For this review, take the finished solid that the model builds, in its own axes (mm). Face numbers are marked on the shaded views. A direction names the side the tool comes from. Round coordinates to 2 decimals unless told otherwise and drop trailing zeros. Write each loop counter-clockwise with the first axis right and the second up, starting at its lowest first coordinate (ties: lowest second). Pieces come first, ordered by that corner, then holes. Notation, with made-up numbers: M -18.5,42.25 L 2.5,42.25 A26 cw 2.5,59.25 Z; hole C -35,-6.5 d7. An arc over 180 degrees is marked long. Answer in a Markdown table with one row per item.
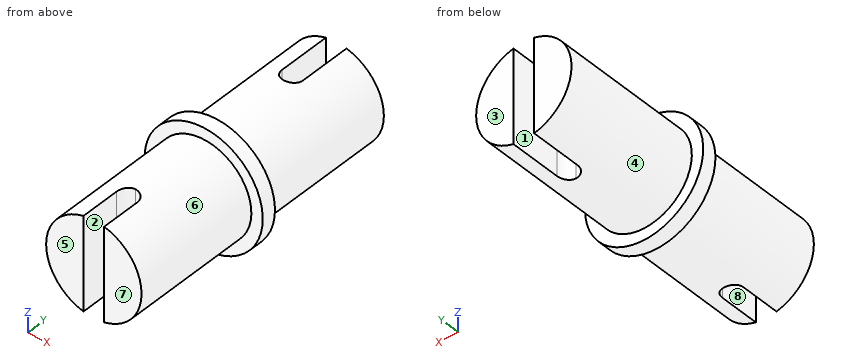
```python
from build123d import *

# Parameters (mm, degrees)
SKETCH2_R            = 2.85
BOSS_EXTRUDE1_DEPTH  = 0.35
SKETCH4_R            = 2.3
BOSS_EXTRUDE2_DEPTH  = 6.9
CUT_EXTRUDE1_START   = -3
CUT_EXTRUDE1_DEPTH   = 3
FILLET1_R            = 0.5
FILLET1_OF_MIRROR1_R = 0.5
CUT_EXTRUDE2_DEPTH   = 0.6


with BuildPart() as part:
    # Sketch2 → Boss-Extrude1 (new body)
    with BuildSketch(Plane(origin=(0, 0, 0), x_dir=(1, 0, 0), z_dir=(0, 1, 0))):
        with Locations(Location((0, 0, 0), (0, 0, 270))):
            Circle(SKETCH2_R)
    boss_extrude1 = extrude(amount=BOSS_EXTRUDE1_DEPTH)

    # Sketch4 → Boss-Extrude2 (add)
    with BuildSketch(Plane(origin=(0, 0.35, 0), x_dir=(1, 0, 0), z_dir=(0, 1, 0))):
        with Locations(Location((0, 0, 0), (0, 0, 90))):
            Circle(SKETCH4_R)
    boss_extrude2 = extrude(amount=BOSS_EXTRUDE2_DEPTH)

    # Sketch5 → Cut-Extrude1 (cut)
    with BuildSketch(Plane(origin=(0, 7.25, 0), x_dir=(1, 0, 0), z_dir=(0, 1, 0)).offset(CUT_EXTRUDE1_START)):
        with BuildLine():
            Line((-0.5, 2.244994432), (-0.5, -2.244994432))
            ThreePointArc((-0.5, -2.244994432), (0, -2.3), (0.5, -2.244994432))
            Line((0.5, -2.244994432), (0.5, 2.244994432))
            ThreePointArc((0.5, 2.244994432), (0, 2.3), (-0.5, 2.244994432))
        make_face()
    cut_extrude1 = extrude(amount=CUT_EXTRUDE1_DEPTH, mode=Mode.SUBTRACT)

    # Fillet1
    fillet1_edges = [part.edges().sort_by_distance(p)[0] for p in [
        (0.5, 4.25, 0),
        (-0.5, 4.25, 0),
    ]]
    fillet(fillet1_edges, radius=FILLET1_R - 0.0001)  # a hair under: the kernel refuses the full size

    # Mirror1: Boss-Extrude1, Boss-Extrude2, Cut-Extrude1 across plane
    add(boss_extrude1.mirror(Plane.ZX))
    add(boss_extrude2.mirror(Plane.ZX))
    add(cut_extrude1.mirror(Plane.ZX), mode=Mode.SUBTRACT)

    # Fillet1 of Mirror1
    fillet1_of_mirror1_edges = [part.edges().sort_by_distance(p)[0] for p in [
        (0.5, -4.25, 0),
        (-0.5, -4.25, 0),
    ]]
    fillet(fillet1_of_mirror1_edges, radius=FILLET1_OF_MIRROR1_R - 0.0001)  # a hair under: the kernel refuses the full size

    # Sketch6 → Cut-Extrude2 (cut)
    with BuildSketch(Plane(origin=(0, -7.25, 0), x_dir=(-1, 0, 0), z_dir=(0, -1, 0))):
        with BuildLine():
            ThreePointArc((0.5, -2.244994432), (2.244994432, 0.5), (-0.5, 2.244994432))
            ThreePointArc((-0.5, 2.244994432), (-2.244994432, -0.5), (0.5, -2.244994432))
        make_face()
    extrude(amount=-CUT_EXTRUDE2_DEPTH, mode=Mode.SUBTRACT)


solid = part.part
```
Q1. For probe 1 along Y at (x, z) = (-1.25, -2.2); probe 2 along X at (y, z) = (-6, -0.45); probe 3 along Z at (x, y) = (-0.1, -2.5), list the stretches that pass through material, from the lowest coordinate up.
Found:
| item | result |
|---|---|
| probe 1 | -0.35 to 0.35 |
| probe 2 | -2.26 to -0.5, 0.5 to 2.26 |
| probe 3 | -2.3 to 2.3 |
Q2. Take a section at B-B (y = 5). State the section outline as (x, z) points (3 decimals).
Found:
| item | result |
|---|---|
| outline | M -0.5,-2.245 L -0.5,2.245 A2.3 ccw Z; M 0.5,-2.245 A2.3 ccw 0.5,2.245 Z |
Q3. Insertion check: P1, Ø1, axis at y = 0.5, z = -2.5, coming from the -X side; P2, Ø2, axis at x = 2, z = 1.5, coming from the +Y side; P3, Ø1.3, axis at y = 5.5, z = -1, coming from the +X side; P4, Ø1, axis at x = 1, y = -4.5, coming from the -Z side (3 decimals). Each pin has a flat end and moves straight along its axis. Give the tip position at first contact, or say it passes through.
Found:
| item | result |
|---|---|
| P1 | x = -2.01 |
| P2 | y = 7.25 |
| P3 | x = 2.27 |
| P4 | z = -2.245 |
Q4. Machinability: for the marked faces 1, 2, 3, 4 and 5, which of the approach directions +Z, -Z, +X, -X, +Y, -Y give a long, thin tool a straight path to every point of the face, cutting with its end or side? Answer none if there is none.
Found:
| item | result |
|---|---|
| face 1 | +Z, -Z, +Y |
| face 2 | +Z, -Z, -Y |
| face 3 | +Z, -Z, +X, -X, +Y |
| face 4 | +Y |
| face 5 | +Z, -Z, +X, -X, -Y |
Q5. Mouldability with a two-part tool opening along X and no side actions: class the marked faces 6, 7 and 8 as +X half, -X half, draft (parallel to the pull), parting line (faces both ways), or undercut.
Found:
| item | result |
|---|---|
| face 6 | parting line |
| face 7 | draft |
| face 8 | undercut |
Q6. Take a section at C-C (x = -0.9). State the section outline as (y, z) points.
Found:
| item | result |
|---|---|
| outline | M -6.65,-2.12 L -0.35,-2.12 L -0.35,-2.7 L 0.35,-2.7 L 0.35,-2.12 L 7.25,-2.12 L 7.25,2.12 L 0.35,2.12 L 0.35,2.7 L -0.35,2.7 L -0.35,2.12 L -6.65,2.12 Z |
Q7. Take a section at D-D (y = 2.5). State the section outline as (x, z) points, then the cut area to 3 significant figures.
Found:
| item | result |
|---|---|
| outline | C 0,0 d4.6 |
| area | 16.6 mm² |
